CAD build for the part. Positions are in the model's coordinates, mm. Face numbers are marked on the shaded views. Round coordinates to 2 decimals unless told otherwise and drop trailing zeros. Loops run counter-clockwise (first coordinate to the right, second up) from the corner with the lowest first, then second, coordinate; pieces in that order, holes last. Notation, with made-up numbers: M 71,36 L 97,36 A21 ccw 97,64 Z; hole C 20.5,72 d8. An arc over 180 degrees is marked long. One line per item, written item: value. Start each with the question number.
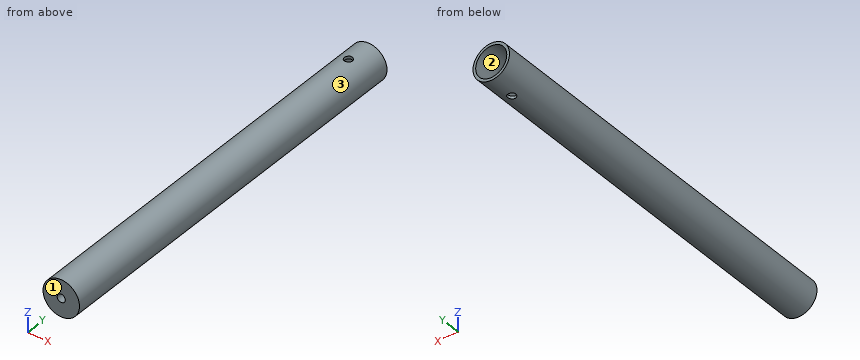
from build123d import *

# Parameters (mm, degrees)
CROQUIS1_R                 = 13.5
SALIENTE_EXTRUIR1_DEPTH    = 300
CROQUIS2_R                 = 3
CORTAR_EXTRUIR1_DEPTH      = 15
CROQUIS4_R                 = 11.5
CORTAR_EXTRUIR4_DEPTH      = 50
CORTAR_EXTRUIR5_DEPTH      = 301.606886149
CORTAR_EXTRUIR5_DEPTH_BACK = 301.606886149
CROQUIS5_R                 = 3


with BuildPart() as part:
    # Croquis1 → Saliente-Extruir1 (new body)
    with BuildSketch(Plane(origin=(0, 0, 0), x_dir=(1, 0, 0), z_dir=(0, 1, 0))):
        with Locations(Location((0, 0, 0), (0, 0, 270))):
            Circle(CROQUIS1_R)
    extrude(amount=SALIENTE_EXTRUIR1_DEPTH)

    # Croquis2 → Cortar-Extruir1 (cut)
    with BuildSketch(Plane.XZ):
        with Locations(Location((0, 0, 0), (0, 0, 270))):
            Circle(CROQUIS2_R)
    extrude(amount=-CORTAR_EXTRUIR1_DEPTH, mode=Mode.SUBTRACT)

    # Croquis4 → Cortar-Extruir4 (cut)
    with BuildSketch(Plane(origin=(0, 300, 0), x_dir=(1, 0, 0), z_dir=(0, 1, 0))):
        with Locations(Location((0, 0, 0), (0, 0, 270))):
            Circle(CROQUIS4_R)
    extrude(amount=-CORTAR_EXTRUIR4_DEPTH, mode=Mode.SUBTRACT)

    # Croquis5 → Cortar-Extruir5 (cut, two sides: drawn at the far end of the back side and taken through both)
    with BuildSketch(Plane.XY.offset(-CORTAR_EXTRUIR5_DEPTH_BACK)):
        with Locations((0, 280)):
            Circle(CROQUIS5_R)
    extrude(amount=CORTAR_EXTRUIR5_DEPTH + CORTAR_EXTRUIR5_DEPTH_BACK, mode=Mode.SUBTRACT)


solid = part.part
(1) Slice it at C-C, the plane z = 0. List the corners of the cut face in (x, y), and give its area (3 significant figures).
(2) Slice it at B-B, the plane y = 280. List the corners of the cut face in (x, z), and give its area (3 significant figures).
(3) Mould opens along X. For the marked faces 1, 2 and 3 say: pulls with the +X half, pulls with the -X half, needs draft (parallel to the pull), parting line crosses it, or undercut.
(4) Slice it at D-D, the plane y = 101. List the corners of the cut face in (x, z), and give its area (3 significant figures).
(5) Probe L1, parallel to Y at x = 0, z = 12.7; L2, parallel to X at y = 7.75, z = 0; L3, parallel to Y at x = -6, z = -8. List the from-to ranges inside material, lowest first.
(6) Flat gauge pins, fed straight in: P1, Ø1, axis at x = 8, y = 122, coming from the +Z side (3 decimals); P2, Ø1.8, axis at x = -1, z = -1, coming from the -Y side; P3, Ø5.5, axis at x = 0, z = 0, coming from the +Y side. Where does each tip first touch, or does it go through?
(7) Slice it at A-A, the plane x = 0. List the corners of the cut face in (y, z).
Check result:
1. outline: M -13.5,0 L -3,0 L -3,15 L 3,15 L 3,0 L 13.5,0 L 13.5,300 L 11.5,300 L 11.5,250 L -11.5,250 L -11.5,300 L -13.5,300 Z
1. area: 6,860 mm^2
2. outline: M -3,-13.16 L -3,-11.1 A11.5 cw -3,11.1 L -3,13.16 A13.5 ccw Z; M 3,-13.16 A13.5 ccw 3,13.16 L 3,11.1 A11.5 cw 3,-11.1 Z
2. area: 133 mm^2
3. face 1: needs draft
3. face 2: undercut
3. face 3: parting line crosses it
4. outline: C 0,0 d27
4. area: 573 mm^2
5. L1: y = 0 to 277, 283 to 300
5. L2: x = -13.5 to -3, 3 to 13.5
5. L3: y = 0 to 250
6. P1: stops at z = 11.225
6. P2: stops at y = 15
6. P3: stops at y = 250
7. outline: M 0,-13.5 L 277,-13.5 L 277,-11.5 L 250,-11.5 L 250,11.5 L 277,11.5 L 277,13.5 L 0,13.5 L 0,3 L 15,3 L 15,-3 L 0,-3 Z; M 283,-13.5 L 300,-13.5 L 300,-11.5 L 283,-11.5 Z; M 283,11.5 L 300,11.5 L 300,13.5 L 283,13.5 Z
